from build123d import *

# Parameters (mm, degrees)
SKETCH1_R           = 75
BOSS_EXTRUDE1_DEPTH = 6.35
SKETCH45_R          = 22.1615
SKETCH45_R_2        = 2.0193
CUT_EXTRUDE36_DEPTH = 107.255929246
FILLET2_R           = 10.16


with BuildPart() as part:
    # Sketch1 → Boss-Extrude1 (new body)
    with BuildSketch(Plane(origin=(0, 0, 0), x_dir=(1, 0, 0), z_dir=(0, 1, 0))):
        with Locations(Location((0, 0, 0), (0, 0, 270))):
            Circle(SKETCH1_R)
    extrude(amount=BOSS_EXTRUDE1_DEPTH)

    # Sketch45 → Cut-Extrude36 (cut, through all)
    with BuildSketch(Plane(origin=(0, 6.35, 0), x_dir=(1, 0, 0), z_dir=(0, 1, 0))):
        with Locations(Location((0, 0, 0), (0, 0, 270))):
            Circle(SKETCH45_R)
        with Locations(Location((-25.4, 25.4, 0), (0, 0, 270))):
            Circle(SKETCH45_R_2)
        with Locations(Location((0, 33.02, 0), (0, 0, 270))):
            Circle(SKETCH45_R_2)
        with Locations(Location((33.02, 0, 0), (0, 0, 270))):
            Circle(SKETCH45_R_2)
        with Locations(Location((0, -33.02, 0), (0, 0, 270))):
            Circle(SKETCH45_R_2)
        with Locations(Location((-33.02, 0, 0), (0, 0, 270))):
            Circle(SKETCH45_R_2)
        with BuildLine():
            Line((-27.903416949, -9.657564215), (-23.915755925, -17.31778977))
            ThreePointArc((-23.915755925, -17.31778977), (-26.616171022, -25.882412255), (-35.180793507, -23.181997158))
            Line((-35.180793507, -23.181997158), (-39.16845453, -15.521771603))
            ThreePointArc((-39.16845453, -15.521771603), (-36.468039434, -6.957149118), (-27.903416949, -9.657564215))
        make_face()
        with BuildLine():
            Line((-28.683948776, -32.276051224), (-51.236957365, -54.829059813))
            ThreePointArc((-51.236957365, -54.829059813), (-54.829059813, -54.829059813), (-54.829059813, -51.236957365))
            Line((-54.829059813, -51.236957365), (-32.276051224, -28.683948776))
            ThreePointArc((-32.276051224, -28.683948776), (-28.683948776, -28.683948776), (-28.683948776, -32.276051224))
        make_face()
        with BuildLine():
            Line((-32.276051224, 28.683948776), (-54.829059813, 51.236957365))
            ThreePointArc((-54.829059813, 51.236957365), (-54.829059813, 54.829059813), (-51.236957365, 54.829059813))
            Line((-51.236957365, 54.829059813), (-28.683948776, 32.276051224))
            ThreePointArc((-28.683948776, 32.276051224), (-28.683948776, 28.683948776), (-32.276051224, 28.683948776))
        make_face()
    extrude(amount=-CUT_EXTRUDE36_DEPTH, mode=Mode.SUBTRACT)

    # Fillet2
    fillet2_edges = [part.edges().sort_by_distance(p)[0] for p in [
        (-51.206535505, 3.175, 54.798637954),
        (-54.798637954, 3.175, 51.206535505),
        (-54.798637954, 3.175, -51.206535505),
        (-51.206535505, 3.175, -54.798637954),
    ]]
    fillet(fillet2_edges, radius=FILLET2_R)


solid = part.part
The model under review builds one solid part; all positions refer to its coordinate system, in mm. A direction names the side the tool comes from. Round coordinates to 2 decimals unless told otherwise and drop trailing zeros. Order: outer loops, then holes, each group sorted by start corner. A loop starts at its lowest first (then second) coordinate and runs counter-clockwise, first axis right, second up. Notation, with made-up numbers: (0.25, -29.75) -> (18.25, -29.75) arc R35 cw to (18.25, 3.25) -> close; hole circle Ø8 at (-4, -32). An arc over 180 degrees is marked (long way). Return JSON: item names as keys, results as strings.
1. Take a section at D-D (x = 65.5). Write out the cut boundary in (y, z), then the cut area to 3 significant figures.
Answer block:
{"outline": "(0, -36.53) -> (6.35, -36.53) -> (6.35, 36.53) -> (0, 36.53) -> close", "area": "464 mm²"}
2. For faces 1 (the face through (-39.415, 3.219, -35.823)), 2 (the face through (-46.078, 3.131, -55.066)), list the 3-axis set-ups (+Z, -Z, +X, -X, +Y, -Y) from which the entire face can be reached by the end or side of a thin tool; tool diameter is ignored.
Answer block:
{"face 1": "+Y, -Y", "face 2": "-X, +Y, -Y"}
3. Take a section at B-B (y = 2.5). Write out the cut boundary in (x, z), then the cut area to 3 significant figures.
Answer block:
{"outline": "(-62.39, -41.62) arc R10.16 ccw to (-46.76, -43.16) -> (-32.28, -28.68) arc R2.54 cw to (-28.68, -32.28) -> (-43.16, -46.76) arc R10.16 ccw to (-41.62, -62.39) arc R75 ccw (long way) to (-41.62, 62.39) arc R10.16 ccw to (-43.16, 46.76) -> (-28.68, 32.28) arc R2.54 cw to (-32.28, 28.68) -> (-46.76, 43.16) arc R10.16 ccw to (-62.39, 41.62) arc R75 ccw to start; hole (-39.17, 15.52) arc R6.35 ccw to (-27.9, 9.66) -> (-23.92, 17.32) arc R6.35 ccw to (-35.18, 23.18) -> close; hole circle Ø4.04 at (-33.02, 0); hole circle Ø4.04 at (-25.4, -25.4); hole circle Ø44.32 at (0, 0); hole circle Ø4.04 at (0, -33.02); hole circle Ø4.04 at (0, 33.02); hole circle Ø4.04 at (33.02, 0)", "area": "15,400 mm²"}
4. Take a section at A-A (x = 33.02). Write out the cut boundary in (y, z).
Answer block:
{"outline": "(0, -67.34) -> (6.35, -67.34) -> (6.35, -2.02) -> (0, -2.02) -> close; (0, 2.02) -> (6.35, 2.02) -> (6.35, 67.34) -> (0, 67.34) -> close"}
5. The part is to be moulded in two halves that separate along X. For faces 3 (the face through (74.966, 3.131, 2.267)), 4 (the face through (-74.997, 3.131, -0.618)), 5 (the face through (18, 6.35, 16)), 6 (the face through (-39.62, 3.22, 36.03)), say which applies: +X half, -X half, draft (parallel to the pull), parting line (faces both ways), or undercut.
Answer block:
{"face 3": "parting line", "face 4": "-X half", "face 5": "draft", "face 6": "undercut"}
6. For L1, parallel to X at y = 2.25, z = -33.02; L2, parallel to Z at x = -41.5, y = 3.5; L3, parallel to X at y = 0.5, z = -33.5, list the stretches that pass through material, from the lowest coordinate up. Write a range as [from, to].
Answer block:
{"L1": "x = [-67.34, -36.61], [-29.43, -2.02], [2.02, 67.34]", "L2": "z = [-62.47, -45.09], [-37.91, 37.91], [45.09, 62.47]", "L3": "x = [-67.1, -37.09], [-29.91, -1.96], [1.96, 67.1]"}
7. Insertion check: P1, Ø2, axis at x = -36.5, y = 3, coming from the +Z side; P2, Ø3, axis at x = -33.02, z = 0, coming from the +Y side; P3, Ø1, axis at x = 53, y = 4.5, coming from the +Z side. Each pin has a flat end and moves straight along its axis. Give the tip position at first contact, or say it passes through.
Answer block:
{"P1": "stops at z = 66.07", "P2": "passes through", "P3": "stops at z = 53.56"}
8. Take a section at C-C (z = -25.4). Write out the cut boundary in (x, y), then the cut area to 3 significant figures.
Answer block:
{"outline": "(-70.57, 0) -> (-27.42, 0) -> (-27.42, 6.35) -> (-70.57, 6.35) -> close; (-23.38, 0) -> (70.57, 0) -> (70.57, 6.35) -> (-23.38, 6.35) -> close", "area": "871 mm²"}
